Check sheet for the modelled part. Datum: model origin and axes. Units: mm. A direction names the side the tool comes from. Coordinates: 2 decimals unless noted, no trailing zeros. Loops run counter-clockwise (first coordinate to the right, second up) from the corner with the lowest first, then second, coordinate; pieces in that order, holes last. Notation, with made-up numbers: (82.5, 11) -> (88.5, 11) arc R36 ccw to (88.5, 46) -> close; hole circle Ø1 at (-26.5, -2.5). An arc over 180 degrees is marked (long way). Use CSV: the item, a comma, the result in double quotes. Start each with the question number.
1. Release check for a two-part mould opening along Y. For faces 6 (the face through (88.72, 88.37, 96.77)), 7 (the face through (38.633, 20.5, 99.695)), 8 (the face through (1.449, 25.756, 125.472)) record: pulls with the +Y half, pulls with the -Y half, needs draft (parallel to the pull), parting line crosses it, or undercut.
2. Sectioned sample at A-A, the plane z = 36.5. Record the cut outline in (x, y).
3. Set-up check for faces 1 (the face through (69, 89, 121.92)), 2 (the face through (38.1, 88, 77)), 3 (the face through (38, 0, 60)), 4 (the face through (89, 50.8, 97)), 5 (the face through (57, 88, 33.02)): record each of +Z, -Z, +X, -X, +Y, -Y from which the full face is reachable in a straight line by a thin tool's end or side.
4. Sectioned sample at B-B, the plane x = 47. Record the cut outline in (y, z).
5. Sectioned sample at D-D, the plane x = 88. Record the cut outline in (y, z).
6. Sectioned sample at C-C, the plane y = 40.5. Record the cut outline in (x, z), and give its area (3 significant figures).
7. Thickness scan on L1, parallel to Z at x = 46, y = 20; L2, parallel to Y at x = 16.5, z = 71; L3, parallel to Z at x = 71.5, y = 87. Record the ranges inside material, lowest first.
8. Gauge pin test, flat ends, axial feed: pin 1 (3 mm diameter, centred on y = 97.5, z = 64, fed in from +X); pin 2 (10 mm diameter, centred on x = 87, z = 68.5, fed in from -Y); pin 3 (2 mm diameter, centred on x = 45, y = 73.5, fed in from +Z); pin 4 (5 mm diameter, centred on y = 21.36, z = 103.57, fed in from +X). Record the tip position at first contact, or that the pin passes through.
```python
from build123d import *

# Parameters (mm, degrees)
F0_W     = 76.2
F0_H     = 50.8
F1_DEPTH = 127
F2_R     = 5.08
F4_D     = 7.9375
F5_W     = 38.1
F5_H     = 88.9
F6_DEPTH = 76.2
F8_DEPTH = 25.4


with BuildPart() as f1:
    # F0 (on Top) → F1 (new body)
    with BuildSketch(Plane.XY):
        with Locations((38.1, 25.4)):
            Rectangle(F0_W, F0_H)
    extrude(amount=F1_DEPTH)

    # F2
    f2_edges = [f1.edges().sort_by_distance(p)[0] for p in [
        (0, 25.4, 127),
        (38.1, 0, 127),
        (76.2, 25.4, 127),
        (38.1, 50.8, 127),
    ]]
    fillet(f2_edges, radius=F2_R)

    # F4 (through all)
    with Locations(Plane(origin=(0, 0, 0), x_dir=(0, -1, 0), z_dir=(-1, 0, 0))):
        with Locations((-21.3607754558, 103.5690684751), (-21.3607754558, 27.3690684751)):
            Hole(F4_D / 2)

    # F5 (on face) → F6 (join)
    with BuildSketch(Plane(origin=(0, 50.8, 0), x_dir=(-1, 0, 0), z_dir=(0, 1, 0))):
        with Locations((-57.15, 77.47)):
            Rectangle(F5_W, F5_H)
    extrude(amount=F6_DEPTH)

    # F7 (on face) → F8 (join)
    with BuildSketch(Plane.YZ.offset(76.2)):
        Polygon((127, 121.92), (50.8, 121.92), (50.8, 72.3118260503), align=None)
    extrude(amount=F8_DEPTH)


solid = f1.part
```
Completed:
1,face 6,"pulls with the +Y half"
1,face 7,"undercut"
1,face 8,"needs draft"
2,outline,"(0, 0) -> (76.2, 0) -> (76.2, 127) -> (38.1, 127) -> (38.1, 50.8) -> (0, 50.8) -> close"
3,face 1,"+Z, +X, -X, +Y"
3,face 2,"+Z, -Z, -X, +Y"
3,face 3,"+Z, -Z, +X, -X, -Y"
3,face 4,"+Z, -Z, +X, -Y"
3,face 5,"-Z, +X, -X, +Y"
4,outline,"(0, 0) -> (50.8, 0) -> (50.8, 33.02) -> (127, 33.02) -> (127, 121.92) -> (50.8, 121.92) arc R5.08 ccw to (45.72, 127) -> (5.08, 127) arc R5.08 ccw to (0, 121.92) -> close; hole circle Ø7.94 at (21.36, 27.37); hole circle Ø7.94 at (21.36, 103.57)"
5,outline,"(50.8, 72.31) -> (127, 121.92) -> (50.8, 121.92) -> close"
6,outline,"(0, 0) -> (76.2, 0) -> (76.2, 121.92) arc R5.08 ccw to (71.12, 127) -> (5.08, 127) arc R5.08 ccw to (0, 121.92) -> close"
6,area,"9,670 mm²"
7,L1,"0 to 23.64, 31.1 to 99.84, 107.3 to 127"
7,L2,"0 to 50.8"
7,L3,"33.02 to 121.92"
8,pin 1,"x = 76.2"
8,pin 2,"y = 50.8"
8,pin 3,"z = 121.92"
8,pin 4,"through"
